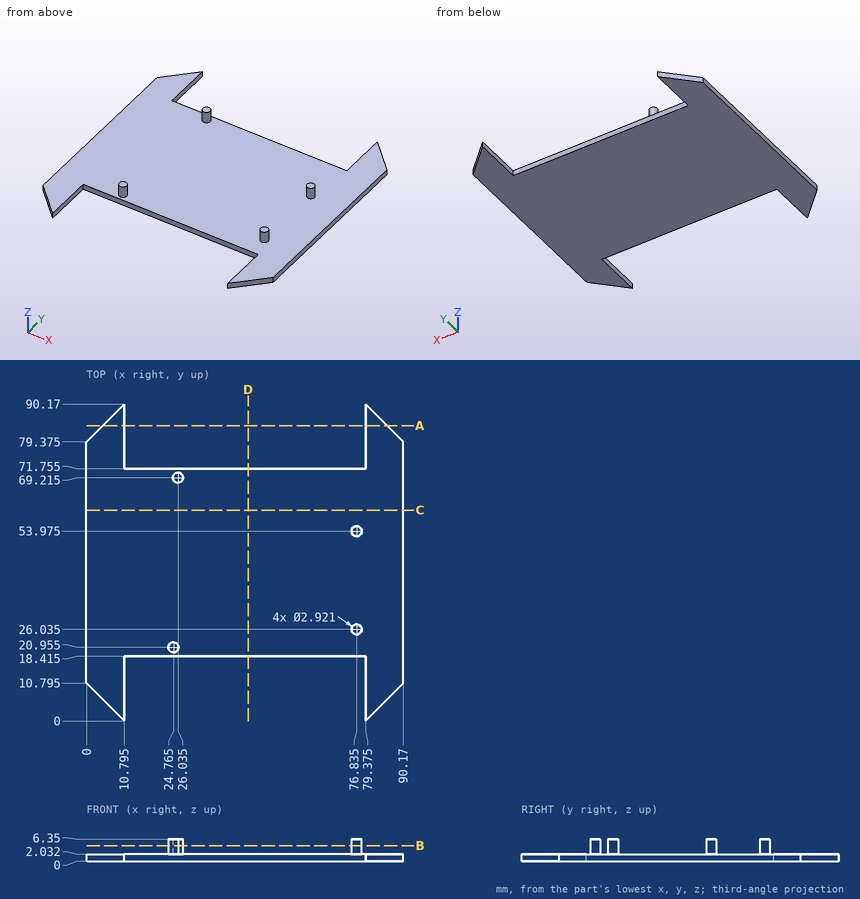
Print and shaded views of the part. All mm, measured from the part's lowest x, y and z. Coordinates: 2 decimals unless noted, no trailing zeros. Loops run counter-clockwise (first coordinate to the right, second up) from the corner with the lowest first, then second, coordinate; pieces in that order, holes last. Notation, with made-up numbers: (77, -29) -> (89, -29) arc R5 cw to (89, -24) -> close; hole circle Ø11 at (35.5, -14). An arc over 180 degrees is marked (long way). Use a Markdown table: item, result. Add a question column.
Item 1: Band-saw the part on D-D on x = 46. Write the cut outline in (y, z) (3 decimals), plus the area to 3 significant figures.
Item 2: Band-saw the part on A-A on y = 84. Write the cut outline in (x, z) (3 decimals).
Item 3: Flat gauge pins, fed straight in: P1, Ø1.6, axis at y = 85, z = 1.5, coming from the +X side (3 decimals); P2, Ø1, axis at x = 64, y = 19.5, coming from the +Z side; P3, Ø0.6, axis at y = 7.5, z = 0.5, coming from the -X side (3 decimals). Where does each tip first touch, or does it go through?
Item 4: Probe probe 1 along Z at (x, y) = (41.5, 51); probe 2 along Y at (x, z) = (25.5, 0.5) (3 decimals); probe 3 along Y at (x, z) = (76.5, 3). List the from-to ranges inside material, lowest first.
Item 5: Band-saw the part on C-C on y = 60. Write the cut outline in (x, z).
Item 6: Band-saw the part on B-B on z = 4.5. Write the cut outline in (x, y) (1 decimal).
Geometry says:
| question | item | result |
|---|---|---|
| 1 | outline | (18.415, 0) -> (71.755, 0) -> (71.755, 2.032) -> (18.415, 2.032) -> close |
| 1 | area | 108 mm² |
| 2 | outline | (4.625, 0) -> (10.795, 0) -> (10.795, 2.032) -> (4.625, 2.032) -> close; (79.375, 0) -> (85.545, 0) -> (85.545, 2.032) -> (79.375, 2.032) -> close |
| 3 | P1 | x = 85.345 |
| 3 | P2 | z = 2.03 |
| 3 | P3 | x = 2.995 |
| 4 | probe 1 | 0 to 2.03 |
| 4 | probe 2 | 18.415 to 71.755 |
| 4 | probe 3 | 24.61 to 27.46, 52.55 to 55.4 |
| 5 | outline | (0, 0) -> (90.17, 0) -> (90.17, 2.03) -> (0, 2.03) -> close |
| 6 | outline | circle Ø2.9 at (24.8, 21); circle Ø2.9 at (26, 69.2); circle Ø2.9 at (76.8, 26); circle Ø2.9 at (76.8, 54) |
